Read the model definition and answer for the solid it produces. Units are mm, in the model's axes. Face numbers are marked on the shaded views. Round coordinates to 2 decimals unless told otherwise and drop trailing zeros. Write each loop counter-clockwise with the first axis right and the second up, starting at its lowest first coordinate (ties: lowest second). Pieces come first, ordered by that corner, then holes. Notation, with made-up numbers: (-10, -19.75) - (25, -19.75) arc R11 ccw to (25, -6.75) - close; hole circle Ø3 at (44, 19.25). An arc over 180 degrees is marked (long way). Answer as CSV lines item,"result". Start each with the question number.
1) Find section D-D on y = 2.25. Determine the outline of the cut face in (x, z), then the cut area to 3 significant figures.
2) Each of these flat-tipped pins is pushed along its axis until it touches: pin 1 (1.1 mm diameter, centred on x = 0, y = 0, fed in from +Z); pin 2 (2 mm diameter, centred on x = 4, z = 1, fed in from -Y); pin 3 (3 mm diameter, centred on y = 2, z = 5.5, fed in from -X); pin 4 (2 mm diameter, centred on x = 5, z = 5.5, fed in from +Y). Where does it stop, or does it pass through?
3) Find section B-B on x = 2.25. Determine the outline of the cut face in (y, z).
4) For a pull along X with two mould halves and no side action, classify the marked faces 1, 2 and 3 as +X half, -X half, draft (parallel to the pull), parting line (faces both ways), or undercut.
5) Consider line 1 along Y through (x, z) = (2.25, 7.75); line 2 along X through (y, z) = (1, 2.5); line 3 along X through (y, z) = (0.5, 4.25). Determine where each line is inside the solid, lowest interval first.
6) Find section C-C on z = 2.5. Determine the outline of the cut face in (x, y).
7) Find section A-A on y = 0. Determine the outline of the cut face in (x, z).
from build123d import *

# Parameters (mm, degrees)
CYLINDER001_R     = 0.88
CYLINDER001_DEPTH = 10
CYLINDER002_R     = 1.75
CYLINDER002_DEPTH = 10
CYLINDER_R        = 2.88
CYLINDER_DEPTH    = 10
CYLINDER003_R     = 4
CYLINDER003_DEPTH = 10


with BuildPart() as filament:
    # Cylinder001 → Cylinder001 (new body)
    with BuildSketch(Plane.XY):
        Circle(CYLINDER001_R)
    extrude(amount=CYLINDER001_DEPTH)


with BuildPart() as screw:
    # Cylinder002 → Cylinder002 (new body)
    with BuildSketch(Plane(origin=(2.25, 0, 0), x_dir=(1, 0, 0), z_dir=(0, 0, 1))):
        Circle(CYLINDER002_R)
    extrude(amount=CYLINDER002_DEPTH)


with BuildPart() as supportfilament:
    # Cylinder → Cylinder (new body)
    with BuildSketch(Plane.XY):
        Circle(CYLINDER_R)
    extrude(amount=CYLINDER_DEPTH)


with BuildPart() as cut001:
    # Cylinder003 → Cylinder003 (new body)
    with BuildSketch(Plane(origin=(2.25, 0, 0), x_dir=(1, 0, 0), z_dir=(0, 0, 1))):
        Circle(CYLINDER003_R)
    extrude(amount=CYLINDER003_DEPTH)

    # Fusion: union SupportFilament
    add(supportfilament.part)

    # Cut: cut Screw
    add(screw.part, mode=Mode.SUBTRACT)

    # Cut001: cut Filament
    add(filament.part, mode=Mode.SUBTRACT)


solid = cut001.part
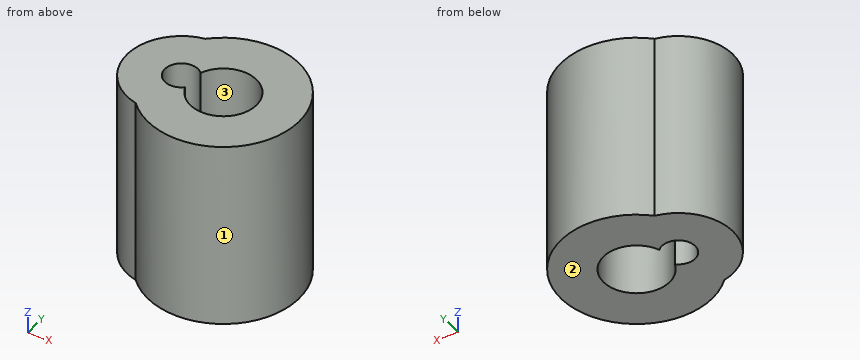
Check values:
1,outline,"(-1.8, 0) - (5.56, 0) - (5.56, 10) - (-1.8, 10) - close"
1,area,"73.5 mm^2"
2,pin 1,"passes through"
2,pin 2,"stops at y = -3.93"
2,pin 3,"stops at x = -2.84"
2,pin 4,"stops at y = 3.6"
3,outline,"(-4, 0) - (-1.75, 0) - (-1.75, 10) - (-4, 10) - close; (1.75, 0) - (4, 0) - (4, 10) - (1.75, 10) - close"
4,face 1,"parting line"
4,face 2,"draft"
4,face 3,"undercut"
5,line 1,"y = -4 to -1.75, 1.75 to 4"
5,line 2,"x = -2.7 to 0.81, 3.69 to 6.12"
5,line 3,"x = -2.84 to -0.72, 3.93 to 6.22"
6,outline,"(-0.59, -2.82) arc R4 ccw (long way) to (-0.59, 2.82) arc R2.88 ccw to start; hole (0.62, -0.63) arc R1.75 ccw (long way) to (0.62, 0.63) arc R0.88 ccw (long way) to start"
7,outline,"(-2.88, 0) - (-0.88, 0) - (-0.88, 10) - (-2.88, 10) - close; (4, 0) - (6.25, 0) - (6.25, 10) - (4, 10) - close"
